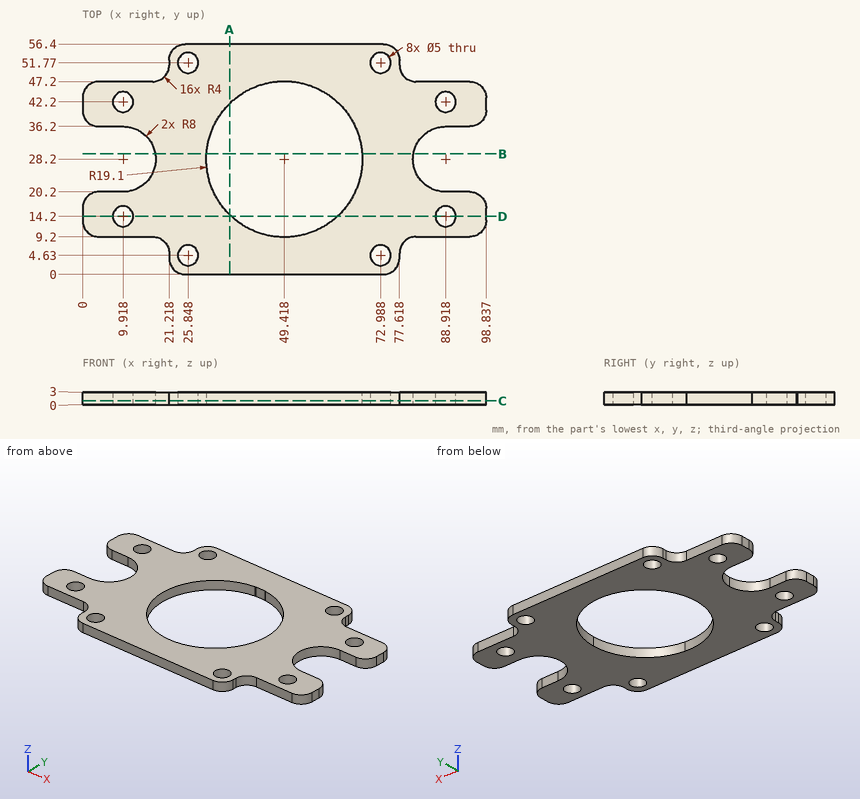
Geometry: see drawing. Coordinates: mm, zero at the bounding-box minimum. Round coordinates to 2 decimals unless told otherwise and drop trailing zeros. Loops run counter-clockwise (first coordinate to the right, second up) from the corner with the lowest first, then second, coordinate; pieces in that order, holes last.
(1) Section query C-C (z = 0.9). Give the number of separate pieces and of enclosed holes in the cut face.
From the geometry:
separate pieces: 1
enclosed holes: 9
(2) Contact query for flat-ended pins moving along their axis: pin 1 Ø0.9 at (x, z) = (7.5, 1.5) entering from -Y; pin 2 Ø6.5 at (x, y) = (88.92, 42.2) entering from -Z; pin 3 Ø1 at (y, z) = (51.5, 1) entering from -X; pin 4 Ø3 at (x, y) = (64, 37.5) entering from +Z. Output: stop coordinate, or through.
From the geometry:
pin 1: stops at y = 9.2
pin 2: stops at z = 0
pin 3: stops at x = 21.21
pin 4: passes through
(3) Section query A-A (x = 36). Output: boundary loops of the cut face in (y, z).
From the geometry:
outline: (0, 0) - (14.61, 0) - (14.61, 3) - (0, 3) - close; (41.79, 0) - (56.4, 0) - (56.4, 3) - (41.79, 3) - close
(4) Section query D-D (y = 14.2). Output: boundary loops of the cut face in (x, z) (1 decimal).
From the geometry:
outline: (0, 0) - (7.4, 0) - (7.4, 3) - (0, 3) - close; (12.4, 0) - (36.4, 0) - (36.4, 3) - (12.4, 3) - close; (62.4, 0) - (86.4, 0) - (86.4, 3) - (62.4, 3) - close; (91.4, 0) - (98.8, 0) - (98.8, 3) - (91.4, 3) - close
(5) Material intervals for probe 1 along X at (y, z) = (28, 0.8) (1 decimal); probe 2 along X at (y, z) = (52, 2.1); probe 3 along X at (y, z) = (40, 2.35) (1 decimal), sorted ascending.
From the geometry:
probe 1: x = 17.9 to 30.3, 68.5 to 80.9
probe 2: x = 21.22 to 23.36, 28.34 to 70.5, 75.48 to 77.62
probe 3: x = 0 to 8.7, 11.1 to 34.4, 64.4 to 87.7, 90.1 to 98.8
(6) Section query B-B (y = 29.5). Output: boundary loops of the cut face in (x, z) (1 decimal).
From the geometry:
outline: (17.8, 0) - (30.4, 0) - (30.4, 3) - (17.8, 3) - close; (68.5, 0) - (81, 0) - (81, 3) - (68.5, 3) - close
